Study the drawing (mm; zero at the part's minimum x, y, z) and answer. Coordinates: 2 decimals unless noted, no trailing zeros. Write each loop counter-clockwise with the first axis right and the second up, starting at its lowest first coordinate (ties: lowest second). Pieces come first, ordered by that corner, then holes. Notation, with made-up numbers: (4.25, -23.75) -> (18.25, -23.75) arc R25 cw to (18.25, 4.25) -> close; hole circle Ø8 at (-12, 75.25). An arc over 180 degrees is marked (long way). Write item = value, one per line. Start each with the question number.
1) Find the intervals of material crossed by line 1 along Z through (x, y) = (31.5, 103) (1 decimal); line 2 along X through (y, z) = (80.5, 32.5); line 3 along Z through (x, y) = (30, 149.5), in increasing order. Write a range as from..to.
2) Flat-ended cylindrical pins translate along their axes: pin 1 Ø5 at (x, y) = (40, 144.5) entering from -Z; pin 2 Ø10 at (y, z) = (90, 17.5) entering from +X; pin 3 Ø8 at (y, z) = (130.5, 32.5) entering from +X. Find the tip coordinate at first contact, or state that the pin passes through.
3) Section B-B (z = 32.5) is taken. Determine the outline of the cut face in (x, y).
4) Section C-C (y = 160) is taken. Determine the outline of the cut face in (x, z), plus the area to 3 significant figures.
5) For a pull along X with two mould halves and no side action, classify the marked faces 1 and 2 as released by +X, released by -X, zero draft, split by the parting line, or undercut.
6) Section A-A (x = 32.5) is taken. Determine the outline of the cut face in (y, z).
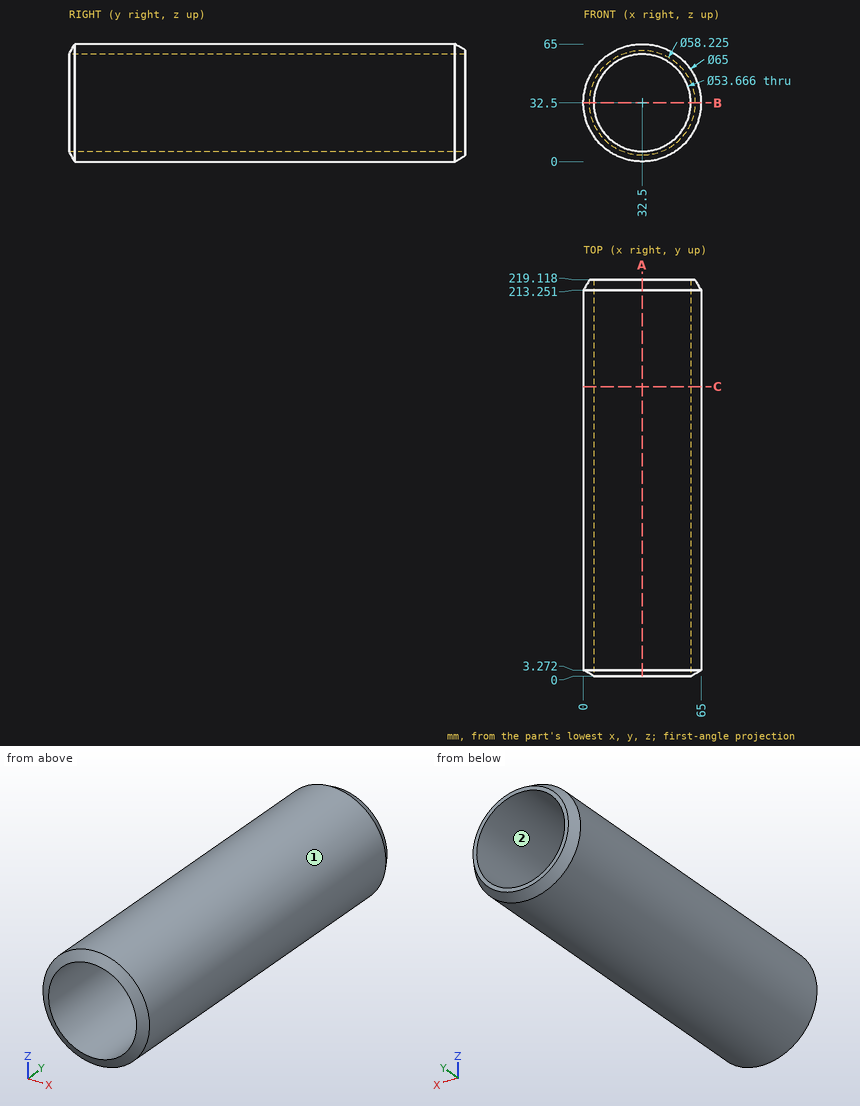
Answer key:
q1.line_1 = 0..5.7, 59.3..65
q1.line_2 = 0..5.67, 59.33..65
q1.line_3 = 0.1..5.78, 59.22..64.9
q2.pin_1 = 0.39
q2.pin_2 = 63.42
q2.pin_3 = 65
q3.outline = (0, 3.27) -> (5.67, 0) -> (5.67, 219.12) -> (3.39, 219.12) -> (0, 213.25) -> close; (59.33, 0) -> (65, 3.27) -> (65, 213.25) -> (61.61, 219.12) -> (59.33, 219.12) -> close
q4.outline = circle Ø65 at (32.5, 32.5); hole circle Ø53.67 at (32.5, 32.5)
q4.area = 1,060 mm^2
q5.face_1 = split by the parting line
q5.face_2 = undercut
q6.outline = (0, 5.67) -> (3.27, 0) -> (213.25, 0) -> (219.12, 3.39) -> (219.12, 5.67) -> close; (0, 59.33) -> (219.12, 59.33) -> (219.12, 61.61) -> (213.25, 65) -> (3.27, 65) -> close
